Geometry: final body of the model. Coordinates: model frame, mm. A direction names the side the tool comes from. Coordinates: 2 decimals unless noted, no trailing zeros. Write each loop counter-clockwise with the first axis right and the second up, starting at its lowest first coordinate (ties: lowest second). Pieces come first, ordered by that corner, then holes. Notation, with made-up numbers: (49, 29.25) -> (100, 29.25) arc R22 cw to (100, 53.25) -> close; hole circle Ø5 at (30.5, -38.5). An arc over 180 degrees is marked (long way). One line per item, written item: value. Start each with the question number.
from build123d import *

# Parameters (mm, degrees)
CROQUIS1_R                   = 3.5
SALIENTE_EXTRUIR1_DEPTH      = 180
SALIENTE_EXTRUIR2_DEPTH      = 8
SALIENTE_EXTRUIR2_DEPTH_BACK = 1
CROQUIS2_R                   = 6
CROQUIS3_R                   = 10
SALIENTE_EXTRUIR3_DEPTH      = 3.5
SALIENTE_EXTRUIR4_START      = -3.5
SALIENTE_EXTRUIR4_DEPTH      = 3.5
CHAFL_N1_SIZE                = 1.5
CHAFL_N1_SIZE2               = 0.866025404
CROQUIS5_R                   = 8
SALIENTE_EXTRUIR5_DEPTH      = 9
CROQUIS6_R                   = 9
SALIENTE_EXTRUIR6_DEPTH      = 2
SALIENTE_EXTRUIR7_START      = -2
SALIENTE_EXTRUIR7_DEPTH      = 2
CROQUIS12_R                  = 4.5
SALIENTE_EXTRUIR11_DEPTH     = 3
CROQUIS13_R                  = 1.8
SALIENTE_EXTRUIR12_DEPTH     = 15
CROQUIS18_W                  = 10
CROQUIS18_H                  = 2
SALIENTE_EXTRUIR16_DEPTH     = 4
SALIENTE_EXTRUIR17_DEPTH     = 6
CORTAR_EXTRUIR3_START        = -4
CORTAR_EXTRUIR3_DEPTH        = 4
SALIENTE_EXTRUIR18_START     = 6
SALIENTE_EXTRUIR18_DEPTH     = 6
REDONDEO7_R                  = 2
REDONDEO8_R                  = 1


with BuildPart() as part:
    # Croquis1 → Saliente-Extruir1 (new body)
    with BuildSketch(Plane.XY):
        with Locations(Location((0, 0, 0), (0, 0, 180))):
            Circle(CROQUIS1_R)
    extrude(amount=SALIENTE_EXTRUIR1_DEPTH)

    # Croquis2 → Saliente-Extruir2 (add, two sides: drawn at the far end of the back side and taken through both)
    with BuildSketch(Plane.XY.offset(180).offset(-SALIENTE_EXTRUIR2_DEPTH_BACK)):
        Circle(CROQUIS2_R)
    extrude(amount=SALIENTE_EXTRUIR2_DEPTH + SALIENTE_EXTRUIR2_DEPTH_BACK)

    # Croquis3 → Saliente-Extruir3 (add)
    with BuildSketch(Plane.XY.offset(188)):
        Circle(CROQUIS3_R)
    extrude(amount=SALIENTE_EXTRUIR3_DEPTH)

    # Croquis4 → Saliente-Extruir4 (add)
    with BuildSketch(Plane.XY.offset(191.5).offset(SALIENTE_EXTRUIR4_START)):
        with BuildLine():
            Line((2.043748165, 9.788927083), (22.095380186, 5.602514639))
            ThreePointArc((22.095380186, 5.602514639), (28.095380186, -0.397485361), (22.095380186, -6.397485361))
            Line((22.095380186, -6.397485361), (2.043748165, -9.788927083))
            ThreePointArc((2.043748165, -9.788927083), (10, 0), (2.043748165, 9.788927083))
        make_face()
    extrude(amount=SALIENTE_EXTRUIR4_DEPTH)

    # Chaflán1
    chafl_n1_edges = [part.edges().sort_by_distance(p)[0] for p in [
        (-6, 0, 179),
    ]]
    chafl_n1_side = [part.faces().sort_by_distance(p)[0] for p in [
        (-5.830294373, 0, 179),
    ]]
    chamfer(chafl_n1_edges, length=CHAFL_N1_SIZE, length2=CHAFL_N1_SIZE2, reference=chafl_n1_side[0])

    # Croquis5 → Saliente-Extruir5 (add)
    with BuildSketch(Plane(origin=(0, 0, 0), x_dir=(-1, 0, 0), z_dir=(0, 0, -1))):
        Circle(CROQUIS5_R)
    extrude(amount=SALIENTE_EXTRUIR5_DEPTH)

    # Croquis6 → Saliente-Extruir6 (add)
    with BuildSketch(Plane(origin=(0, 0, -9), x_dir=(-1, 0, 0), z_dir=(0, 0, -1))):
        Circle(CROQUIS6_R)
    extrude(amount=SALIENTE_EXTRUIR6_DEPTH)

    # Croquis7 → Saliente-Extruir7 (add)
    with BuildSketch(Plane(origin=(0, 0, -11), x_dir=(-1, 0, 0), z_dir=(0, 0, -1)).offset(SALIENTE_EXTRUIR7_START)):
        with BuildLine():
            Line((-5, -7.483314774), (-5, -11.483314774))
            Line((-5, -11.483314774), (5, -11.483314774))
            Line((5, -11.483314774), (5, -7.483314774))
            ThreePointArc((5, -7.483314774), (0, -9), (-5, -7.483314774))
        make_face()
    extrude(amount=SALIENTE_EXTRUIR7_DEPTH)

    # Croquis12 → Saliente-Extruir11 (add)
    with BuildSketch(Plane.XY.offset(191.5)):
        with Locations((22.095380186, -0.397485361)):
            Circle(CROQUIS12_R)
    extrude(amount=SALIENTE_EXTRUIR11_DEPTH)

    # Croquis13 → Saliente-Extruir12 (add)
    with BuildSketch(Plane.XY.offset(194.5)):
        with Locations((22.095380186, -0.397485361)):
            Circle(CROQUIS13_R)
    extrude(amount=SALIENTE_EXTRUIR12_DEPTH)

    # Croquis18 → Saliente-Extruir16 (add)
    with BuildSketch(Plane(origin=(0, 0, -11), x_dir=(-1, 0, 0), z_dir=(0, 0, -1))):
        with Locations((0, -10.483314774)):
            Rectangle(CROQUIS18_W, CROQUIS18_H)
    extrude(amount=SALIENTE_EXTRUIR16_DEPTH)

    # Croquis19 → Saliente-Extruir17 (add)
    with BuildSketch(Plane(origin=(0, 0, -15), x_dir=(-1, 0, 0), z_dir=(0, 0, -1))):
        with BuildLine():
            Line((14.328458937, 0), (16.318610319, 0))
            ThreePointArc((16.318610319, 0), (0, -12.235237964), (-16.318610319, 0))
            Line((-16.318610319, 0), (-14.328458937, 0))
            ThreePointArc((-14.328458937, 0), (0, -10.335161566), (14.328458937, 0))
        make_face()
    extrude(amount=SALIENTE_EXTRUIR17_DEPTH)

    # Croquis20 → Cortar-Extruir3 (cut)
    with BuildSketch(Plane(origin=(0, 0, -15), x_dir=(-1, 0, 0), z_dir=(0, 0, -1)).offset(CORTAR_EXTRUIR3_START)):
        with BuildLine():
            Line((5, -9.483314774), (-5, -9.483314774))
            ThreePointArc((-5, -9.483314774), (0, -10.335161566), (5, -9.483314774))
        make_face()
    extrude(amount=CORTAR_EXTRUIR3_DEPTH, mode=Mode.SUBTRACT)

    # Croquis21 → Saliente-Extruir18 (add)
    with BuildSketch(Plane.XY.offset(-15).offset(SALIENTE_EXTRUIR18_START)):
        with BuildLine():
            Line((5, -11.483314774), (-5, -11.483314774))
            ThreePointArc((-5, -11.483314774), (0, -12.235237964), (5, -11.483314774))
        make_face()
    extrude(amount=-SALIENTE_EXTRUIR18_DEPTH)

    # Redondeo7
    redondeo7_edges = [part.edges().sort_by_distance(p)[0] for p in [
        (0, -12.235237964, -9),
        (0, -10.335161566, -11),
    ]]
    fillet(redondeo7_edges, radius=REDONDEO7_R)

    # Redondeo8
    # the kernel refuses this fillet: 1 mm, written as the material it takes off along each edge
    with BuildSketch(Plane(origin=(-16.318610319, 0, -11.409775172), x_dir=(0.3205749609840578, -0.9472231492051225, 0), z_dir=(0, 0, -1))) as redondeo8_piece_1:
        with BuildLine():
            CenterArc((1.393851992, -0.99910758), REDONDEO8_R, 87.579224192, 111.118475452)
            Line((0.446628843, -1.319682541), (0, 0))
            ThreePointArc((0, 0), (0.718044966, 0.015171139), (1.436089931, 0))
        make_face()
    extrude(amount=13.180449656, mode=Mode.SUBTRACT)
    with BuildSketch(Plane(origin=(-14.328458937, 0, -13.239980297), x_dir=(0.3368909660560179, -0.9415436670648064, 0), z_dir=(0, 0, -1))) as redondeo8_piece_2:
        with BuildLine():
            CenterArc((0.704369772, 0.999745128), REDONDEO8_R, 199.687567709, 69.018809156)
            Line((-0.237173895, 0.662854162), (0, 0))
            ThreePointArc((0, 0), (0.340896854, 0.003848545), (0.681793707, 0))
        make_face()
    extrude(amount=9.520039406, mode=Mode.SUBTRACT)
    with BuildSketch(Plane(origin=(16.318610319, 0, -11.409775172), x_dir=(-0.3205749609840585, -0.9472231492051224, 0), z_dir=(0, 0, -1))) as redondeo8_piece_3:
        with BuildLine():
            CenterArc((1.393851992, 0.99910758), REDONDEO8_R, 161.302300356, 111.118475452)
            Line((0.446628843, 1.319682541), (0, 0))
            ThreePointArc((0, 0), (0.718044966, -0.015171139), (1.436089931, 0))
        make_face()
    extrude(amount=13.180449656, mode=Mode.SUBTRACT)
    with BuildSketch(Plane(origin=(14.328458937, 0, -13.239980297), x_dir=(-0.33689096605601593, -0.9415436670648072, 0), z_dir=(0, 0, -1))) as redondeo8_piece_4:
        with BuildLine():
            CenterArc((0.704369772, -0.999745128), REDONDEO8_R, 91.293623135, 69.018809156)
            Line((-0.237173895, -0.662854162), (0, 0))
            ThreePointArc((0, 0), (0.340896854, -0.003848545), (0.681793707, 0))
        make_face()
    extrude(amount=9.520039406, mode=Mode.SUBTRACT)


solid = part.part
Q1. Access query for faces 1 (the cylindrical face through (26.252, -2.121, 192.979)), 2 (the cylindrical face through (1.73, -7.81, -4.44)), 3 (the flat face through (11, -6, -15)). Directions: +Z, -Z, +X, -X, +Y, -Y. A direction counts if a zero-diameter tool reaches every point of the face in a straight line with its end or side. Return the directions, or none.
Q2. First-contact query: P1, Ø10, axis at x = 1.5, y = 0, coming from the -Z side; P2, Ø1.2, axis at y = -9.5, z = -10.5, coming from the -X side; P3, Ø13, axis at x = 2.5, y = 3.5, coming from the +Z side; P4, Ø1.5, axis at x = 14, y = -10, coming from the -Z side. Flat tips, straight axial feed; report the tip coordinate or a pass-through.
Q3. Cut plane B-B on z = 35.5. Output: boundary loops of the cut face in (x, y), and give its area (3 significant figures).
Q4. Draft query along Z for faces 4 (the flat face through (0, 0, -11)), 5 (the flat face through (-3, -8, -9)), 6 (the flat face through (5, 0, 191.5)), 7 (the cylindrical face through (-3.233, 1.341, 88.247)). Return one class per face: pulls with the +Z half, pulls with the -Z half, needs draft (parallel to the pull), parting line crosses it, or undercut.
Q5. Cut plane A-A on x = 0. Output: boundary loops of the cut face in (y, z).
Q6. Line query: L1, parallel to Z at x = -2, y = 7.5; L2, parallel to Z at x = -4, y = -0.75; L3, parallel to Z at x = 26, y = -2.5. Output: solid intervals per line, ascending. Write a range as from..to.
Solution:
1. face 1: +Z
1. face 2: none
1. face 3: +X, +Y, -Y
2. P1: z = -11
2. P2: x = -5
2. P3: z = 191.5
2. P4: through
3. outline: circle Ø7 at (0, 0)
3. area: 38.5 mm²
4. face 4: pulls with the -Z half
4. face 5: undercut
4. face 6: pulls with the +Z half
4. face 7: undercut
5. outline: (-12.24, -21) -> (-10.34, -21) -> (-10.34, -13) arc R2 cw to (-8.34, -11) -> (9, -11) -> (9, -9) -> (8, -9) -> (8, 0) -> (3.5, 0) -> (3.5, 179) -> (4.5, 179) -> (6, 179.87) -> (6, 188) -> (10, 188) -> (10, 191.5) -> (-10, 191.5) -> (-10, 188) -> (-6, 188) -> (-6, 179.87) -> (-4.5, 179) -> (-3.5, 179) -> (-3.5, 0) -> (-8, 0) -> (-8, -9) -> (-10.24, -9) arc R2 ccw to (-12.24, -11) -> close
6. L1: -11..0, 188..191.5
6. L2: -11..0, 179..191.5
6. L3: 188..194.5
